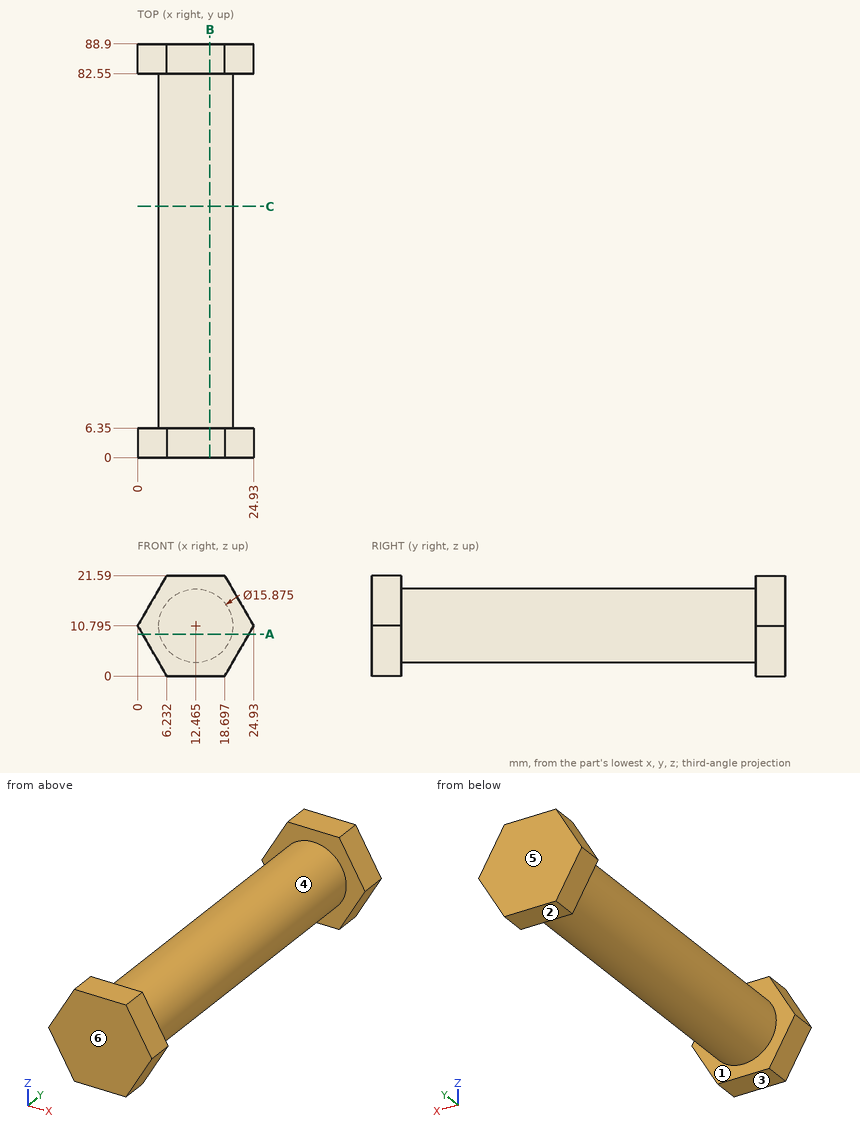
Design review of the part shown in the three views and the two pictorial views. Dimensions are in mm from the part's minimum x, y and z. A direction names the side the tool comes from. Round coordinates to 2 decimals unless told otherwise and drop trailing zeros. Write each loop counter-clockwise with the first axis right and the second up, starting at its lowest first coordinate (ties: lowest second). Pieces come first, ordered by that corner, then holes.
Item 1: We need section B-B on x = 15.5. Write out the cut boundary in (y, z), and give its area (3 significant figures).
Item 2: For the marked faces 1 and 2, list the 3-axis set-ups (+Z, -Z, +X, -X, +Y, -Y) from which the entire face can be reached by the end or side of a thin tool; tool diameter is ignored.
Item 3: Clearance check with flat-ended pins moving along their axes: pin 1 Ø12 at (y, z) = (65, 2.5) entering from -X; pin 2 Ø4 at (y, z) = (13.5, 11) entering from +X; pin 3 Ø10 at (x, y) = (6.5, 31) entering from +Z. State where each tip first meets the part, or that it passes through.
Item 4: The part is to be moulded in two halves that separate along Y. For the marked faces 3, 4, 5 and 6, say which applies: +Y half, -Y half, draft (parallel to the pull), parting line (faces both ways), or undercut.
Item 5: For probe 1 along Y at (x, z) = (18, 20.25); probe 2 along Z at (x, y) = (12, 75); probe 3 along Z at (x, y) = (16.5, 79.5), list the stretches that pass through material, from the lowest coordinate up.
Item 6: We need section C-C on y = 54. Write out the cut boundary in (x, z) (1 decimal).
Item 7: We need section A-A on z = 9. Write out the cut boundary in (x, y), and give its area (3 significant figures).
Returned:
1. outline: (0, 0) - (6.35, 0) - (6.35, 3.46) - (82.55, 3.46) - (82.55, 0) - (88.9, 0) - (88.9, 21.59) - (82.55, 21.59) - (82.55, 18.13) - (6.35, 18.13) - (6.35, 21.59) - (0, 21.59) - close
1. area: 1,390 mm2
2. face 1: none
2. face 2: -Z, +X, -X, +Y, -Y
3. pin 1: stops at x = 4.87
3. pin 2: stops at x = 20.4
3. pin 3: stops at z = 18.67
4. face 3: draft
4. face 4: undercut
4. face 5: +Y half
4. face 6: -Y half
5. probe 1: y = 0 to 6.35, 82.55 to 88.9
5. probe 2: z = 2.87 to 18.72
5. probe 3: z = 3.96 to 17.63
6. outline: circle Ø15.9 at (12.5, 10.8)
7. outline: (1.04, 0) - (23.89, 0) - (23.89, 6.35) - (20.2, 6.35) - (20.2, 82.55) - (23.89, 82.55) - (23.89, 88.9) - (1.04, 88.9) - (1.04, 82.55) - (4.73, 82.55) - (4.73, 6.35) - (1.04, 6.35) - close
7. area: 1,470 mm2
